Can you work these out from the model? Positions are in its coordinate system, mm. Face numbers are marked on the shaded views. A direction names the side the tool comes from. Give positions to 0.01 mm unless a question says otherwise; leave off trailing zeros. Loops run counter-clockwise (first coordinate to the right, second up) from the corner with the lowest first, then second, coordinate; pieces in that order, holes last.
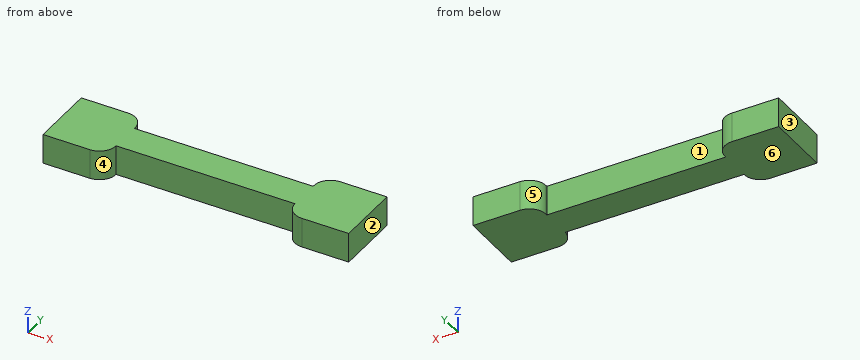
from build123d import *

# Parameters (mm, degrees)
F1_DEPTH = 25.4


with BuildPart() as f1:
    # F0 (on Top) → F1 (new body)
    with BuildSketch(Plane.XY):
        Polygon((-76.211855, 18.343313), (-76.211855, 17.691907), (-76.211855, -8.345137), (0, -8.345137), (0, 8.345137), (0, 18.343313), align=None)
        with BuildLine():
            Line((-76.211855, -8.345137), (-76.211855, 17.691907))
            Line((-76.211855, 17.691907), (-76.211855, 18.343313))
            Line((-76.211855, 18.343313), (-76.211855, 19.464858))
            ThreePointArc((-76.211855, 19.464858), (-80.35492, 29.467103), (-90.357166, 33.610169))
            Line((-90.357166, 33.610169), (-130.292863, 33.610169))
            Line((-130.292863, 33.610169), (-130.292863, -22.490447))
            Line((-130.292863, -22.490447), (-90.357166, -22.490447))
            ThreePointArc((-90.357166, -22.490447), (-80.35492, -18.347382), (-76.211855, -8.345137))
        make_face()
    extrude(amount=F1_DEPTH)

    # F2: F1 across face


with BuildPart() as f1_1:
    add(f1.part)
    add(f1.part.mirror(Plane(origin=(0, 4.999088, 12.7), x_dir=(0, 1, 0), z_dir=(1, 0, 0))))


solid = f1_1.part
(1) Suppose I cut it at D-D on y = 25.5. List the corners of the cut face in (x, z) for me.
Returned:
outline: (-130.29, 0) - (-77.56, 0) - (-77.56, 25.4) - (-130.29, 25.4) - close; (77.56, 0) - (130.29, 0) - (130.29, 25.4) - (77.56, 25.4) - close
(2) Which directions (+Z, -Z, +X, -X, +Y, -Y) give clear straight access to the entire face, cutting with the end or side of a thin tool? Please do the marked faces 4, 5 and 6.
Returned:
face 4: +Z, -Z, -Y
face 5: +Z, -Z, +Y
face 6: -Z, +X, -X, +Y, -Y
(3) Suppose I cut it at A-A on y = -15.5. List the corners of the cut face in (x, z) for me.
Returned:
outline: (-130.29, 0) - (-78.15, 0) - (-78.15, 25.4) - (-130.29, 25.4) - close; (78.15, 0) - (130.29, 0) - (130.29, 25.4) - (78.15, 25.4) - close
(4) Will this pin go through, and if not, where does the flat tip stop? P1, Ø10, axis at x = -37.5, z = 8, coming from the +Y side.
Returned:
P1: stops at y = 18.34
(5) Suppose I cut it at C-C on x = 42. List the corners of the cut face in (y, z) for me, plus the area to 3 significant figures.
Returned:
outline: (-8.35, 0) - (18.34, 0) - (18.34, 25.4) - (-8.35, 25.4) - close
area: 678 mm2
(6) Thinking about a two-plate mould opening in X: for the marked faces 1, 2 and 3, which applies, pulls with the +X half, pulls with the -X half, needs draft (parallel to the pull), parting line crosses it, or undercut?
Returned:
face 1: undercut
face 2: pulls with the +X half
face 3: pulls with the -X half
(7) Please list where these lines run through material, in increasing order: probe 1 along Y at (x, z) = (-17, 12.25); probe 2 along X at (y, z) = (29, 21); probe 3 along X at (y, z) = (31, 13).
Returned:
probe 1: y = -8.35 to 18.34
probe 2: x = -130.29 to -79.91, 79.91 to 130.29
probe 3: x = -130.29 to -82.17, 82.17 to 130.29
(8) Suppose I cut it at B-B on z = 5.5. List the corners of the cut face in (x, y) for me.
Returned:
outline: (-130.29, -22.49) - (-90.36, -22.49) arc R14.15 ccw to (-76.21, -8.35) - (76.21, -8.35) arc R14.15 ccw to (90.36, -22.49) - (130.29, -22.49) - (130.29, 33.61) - (90.36, 33.61) arc R14.15 ccw to (76.21, 19.46) - (76.21, 18.34) - (-76.21, 18.34) - (-76.21, 19.46) arc R14.15 ccw to (-90.36, 33.61) - (-130.29, 33.61) - close
